Input: part model. Units: mm. Frame: model coordinates. A direction names the side the tool comes from. Coordinates: 2 decimals unless noted, no trailing zeros. Order: outer loops, then holes, each group sorted by start corner. A loop starts at its lowest first (then second) coordinate and runs counter-clockwise, first axis right, second up. Notation, with made-up numbers: (49, 81.25) -> (76, 81.25) arc R18 ccw to (76, 110.25) -> close; hole circle Ø9 at (1, 85.25). An arc over 180 degrees is marked (long way). One line per question, with ' | ' between items.
```python
from build123d import *

# Parameters (mm, degrees)
BOSS_EXTRUDE1_DEPTH = 25
CHAMFER2_SIZE       = 10
HOLE1_D             = 15
CHAMFER3_SIZE       = 1
HOLE2_D             = 10
CHAMFER4_SIZE       = 1
CHAMFER5_SIZE       = 1


with BuildPart() as part:
    # Sketch1 → Boss-Extrude1 (new, symmetric)
    with BuildSketch(Plane.XY):
        Polygon((-55, -6.5), (-55, 7.5), (-25, 7.5), (-25, 15), (25, 15), (25, 7.5), (55, 7.5), (55, -6.5), (54, -7.5), (30, -7.5), (30, -14), (29, -15), (-29, -15), (-30, -14), (-30, -7.5), (-54, -7.5), align=None)
    extrude(amount=BOSS_EXTRUDE1_DEPTH, both=True)

    # Chamfer2
    # the kernel refuses this chamfer: 10 mm, written as the material it adds along each edge
    with BuildSketch(Plane(origin=(25, 7.5, 25), x_dir=(0.9996219169112968, -0.027495876610586403, 0), z_dir=(0, 0, -1))) as chamfer2_piece_1_section:
        Polygon((CHAMFER2_SIZE * 0.999621916911, -CHAMFER2_SIZE * 0.0274958766106), (-CHAMFER2_SIZE * 0.0274958766106, -CHAMFER2_SIZE * 0.999621916911), (0, 0), align=None)
    chamfer2_piece_1 = extrude(amount=50, mode=Mode.PRIVATE)
    chamfer2_piece_1 = split(chamfer2_piece_1, bisect_by=Plane(origin=(28.519591102, 15, 0), z_dir=(0, -1, 0)), keep=Keep.TOP, mode=Mode.PRIVATE)
    add(chamfer2_piece_1)
    with BuildSketch(Plane(origin=(-25, 7.5, 25), x_dir=(0.027495876610586317, 0.9996219169112968, 0), z_dir=(0, 0, -1))) as chamfer2_piece_2_section:
        Polygon((CHAMFER2_SIZE * 0.999621916911, -CHAMFER2_SIZE * 0.0274958766106), (-CHAMFER2_SIZE * 0.0274958766106, -CHAMFER2_SIZE * 0.999621916911), (0, 0), align=None)
    chamfer2_piece_2 = extrude(amount=50, mode=Mode.PRIVATE)
    chamfer2_piece_2 = split(chamfer2_piece_2, bisect_by=Plane(origin=(-28.519591102, 15, 0), z_dir=(0, -1, 0)), keep=Keep.TOP, mode=Mode.PRIVATE)
    add(chamfer2_piece_2)

    # Hole1 (through all)
    with Locations(Plane.XY.offset(25)):
        with Locations((0, 0)):
            Hole(HOLE1_D / 2)

    # Chamfer3
    chamfer3_edges = [part.edges().sort_by_distance(p)[0] for p in [
        (7.5, 0, 25),
        (7.5, 0, -25),
    ]]
    chamfer(chamfer3_edges, length=CHAMFER3_SIZE)

    # Hole2 (through all)
    with Locations(Plane(origin=(0, 7.5, 0), x_dir=(1, 0, 0), z_dir=(0, 1, 0))):
        with Locations((42.5, 15), (42.5, -15)):
            hole2 = Hole(HOLE2_D / 2)

    # Chamfer4
    chamfer4_edges = [part.edges().sort_by_distance(p)[0] for p in [
        (47.5, 7.5, 15),
        (47.5, -7.5, 15),
        (47.5, 7.5, -15),
        (47.5, -7.5, -15),
    ]]
    chamfer(chamfer4_edges, length=CHAMFER4_SIZE)

    # Mirror5: Hole2 across plane
    add(hole2.mirror(Plane(origin=(0, 0, 0), x_dir=(0, 0, 1), z_dir=(1, 0, 0))), mode=Mode.SUBTRACT)

    # Chamfer5
    chamfer5_edges = [part.edges().sort_by_distance(p)[0] for p in [
        (-47.5, 7.5, 15),
        (-47.5, -7.5, 15),
        (-47.5, 7.5, -15),
        (-47.5, -7.5, -15),
    ]]
    chamfer(chamfer5_edges, length=CHAMFER5_SIZE)


solid = part.part
```
1. Mould query, pull axis Z, two halves, no side actions, for faces 5 (the face through (-47.495, -0.091, -15.22)), 6 (the face through (0, -10, -25)), 7 (the face through (55, 1, 0)), 8 (the face through (47.495, -0.091, 14.78)). Classes: released by +Z, released by -Z, zero draft, split by the parting line, or undercut.
Recorded:
face 5: undercut | face 6: released by -Z | face 7: zero draft | face 8: undercut
2. Access query for faces 1 (the face through (-42, -7.5, 0)), 2 (the face through (42, -7.5, 0)), 3 (the face through (-45, 7.5, 0)), 4 (the face through (45, 7.5, 0)). Directions: +Z, -Z, +X, -X, +Y, -Y. A direction counts if a zero-diameter tool reaches every point of the face in a straight line with its end or side. Return the directions, or none.
Recorded:
face 1: +Z, -Z, -X, -Y | face 2: +Z, -Z, +X, -Y | face 3: +Z, -Z, -X, +Y | face 4: +Z, -Z, +X, +Y
3. Pin query (flat end, axial travel): pin 1 Ø7 at (x, z) = (-42.5, 4.5) entering from -Y; pin 2 Ø6 at (x, z) = (40.5, 6) entering from +Y; pin 3 Ø3 at (y, z) = (-11, 11.5) entering from +X; pin 4 Ø10 at (y, z) = (12, -16.5) entering from -X. Return the tip coordinate at first contact, or that it passes through.
Recorded:
pin 1: stops at y = -7.5 | pin 2: stops at y = 7.5 | pin 3: stops at x = 30 | pin 4: stops at x = -55
4. Cut plane A-A, the plane z = 15. State how many separate pieces and enclosed holes the cut face has, and give its area (3 significant figures).
Recorded:
separate pieces: 3 | enclosed holes: 1 | area: 2,090 mm^2
5. Cut plane B-B, the plane x = 0. Return loops of the section in (y, z).
Recorded:
outline: (-15, -25) -> (-8.5, -25) -> (-7.5, -24) -> (-7.5, 24) -> (-8.5, 25) -> (-15, 25) -> close; (7.5, -24) -> (8.5, -25) -> (15, -25) -> (15, 25) -> (8.5, 25) -> (7.5, 24) -> close
6. Ray query, line 1 (Z direction, x = 42.5, y = 0.25); line 2 (Y direction, x = 0, z = -6); line 3 (Y direction, x = 34, z = -19). Return the intervals inside material, ascending. Write a range as [from, to].
Recorded:
line 1: z = [-25, -20], [-10, 10], [20, 25] | line 2: y = [-15, -7.5], [7.5, 15] | line 3: y = [-7.5, 8.5]
7. Cut plane C-C, the plane y = 0. Return loops of the section in (x, z), and give its area (3 significant figures).
Recorded:
outline: (-55, -25) -> (-8.5, -25) -> (-7.5, -24) -> (-7.5, 24) -> (-8.5, 25) -> (-55, 25) -> close; (7.5, -24) -> (8.5, -25) -> (55, -25) -> (55, 25) -> (8.5, 25) -> (7.5, 24) -> close; hole circle Ø10 at (-42.5, -15); hole circle Ø10 at (-42.5, 15); hole circle Ø10 at (42.5, -15); hole circle Ø10 at (42.5, 15) | area: 4,430 mm^2
8. Cut plane D-D, the plane x = -42.5. Return loops of the section in (y, z).
Recorded:
outline: (-7.5, -25) -> (7.5, -25) -> (7.5, -21) -> (6.5, -20) -> (-6.5, -20) -> (-7.5, -21) -> close; (-7.5, -9) -> (-6.5, -10) -> (6.5, -10) -> (7.5, -9) -> (7.5, 9) -> (6.5, 10) -> (-6.5, 10) -> (-7.5, 9) -> close; (-7.5, 21) -> (-6.5, 20) -> (6.5, 20) -> (7.5, 21) -> (7.5, 25) -> (-7.5, 25) -> close
